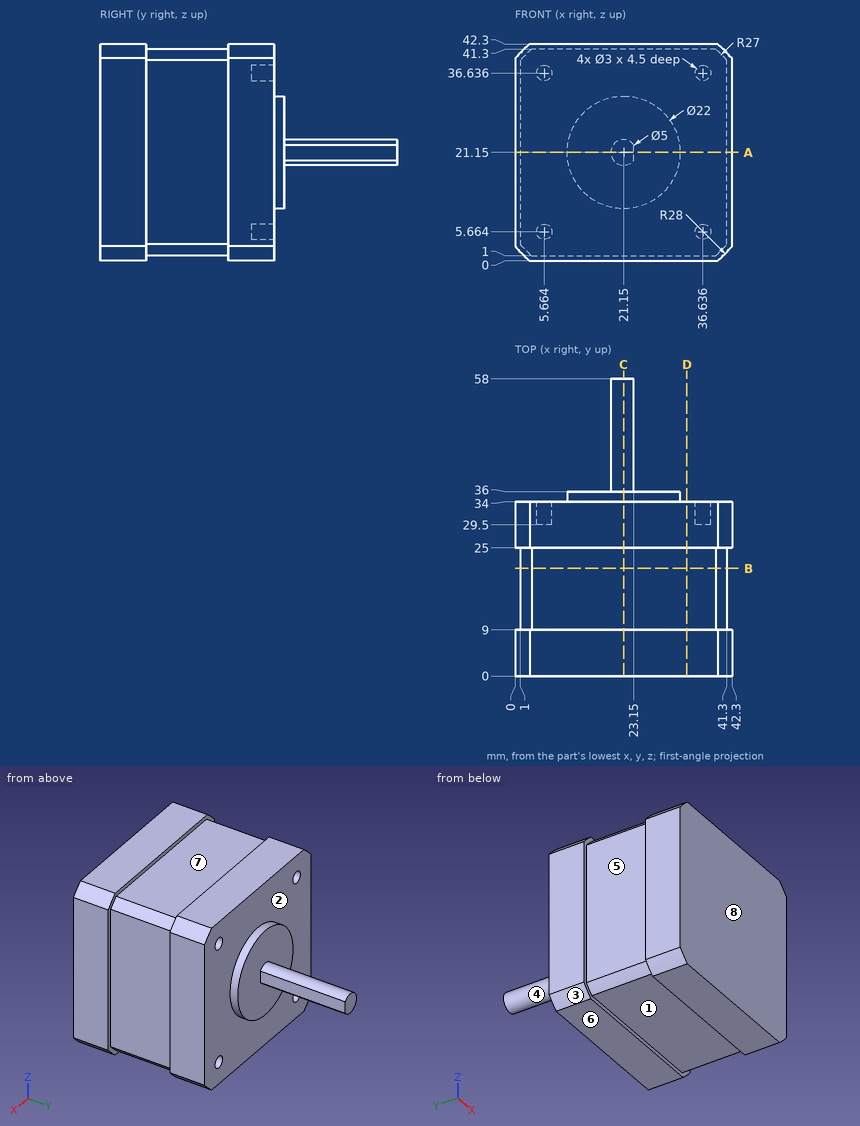
Job drawing, mm, ordinate dimensions from the low corner. One solid piece. A direction names the side the tool comes from. Give positions to 0.01 mm unless a question says otherwise; leave off trailing zeros. Loops run counter-clockwise (first coordinate to the right, second up) from the corner with the lowest first, then second, coordinate; pieces in that order, holes last.
Item 1: Slice it at D-D, the plane x = 33.5. List the corners of the cut face in (y, z), and give its area (3 significant figures).
Answers follow:
outline: (0, 0) - (9, 0) - (9, 1) - (25, 1) - (25, 0) - (34, 0) - (34, 42.3) - (25, 42.3) - (25, 41.3) - (9, 41.3) - (9, 42.3) - (0, 42.3) - close
area: 1,410 mm2
Item 2: Which spindle directions (+Z, -Z, +X, -X, +Y, -Y) get a long thin tool onto all of the face, cutting with end or side? Do the marked faces 4, 5, 6, 7 and 8. Say none if no direction does.
Answers follow:
face 4: +Y
face 5: +Z, -Z, -X
face 6: -Z, +X, -X, +Y, -Y
face 7: +Z, +X, -X
face 8: +Z, -Z, +X, -X, -Y
Item 3: Flat gauge pins, fed straight in: pin 1 (0.9 mm diameter, centred on x = 6, z = 5, fed in from +Y); pin 2 (3.5 mm diameter, centred on x = 36.64, z = 5.66, fed in from +Y); pin 3 (2.5 mm diameter, centred on y = 45.5, z = 21.5, fed in from +X). Where does each tip first touch, or does it go through?
Answers follow:
pin 1: stops at y = 29.5
pin 2: stops at y = 34
pin 3: stops at x = 23.15
Item 4: Drill centre lines: line 1 (Y direction, x = 24.5, z = 38); line 2 (X direction, y = 33.5, z = 5); line 3 (X direction, y = 11, z = 33.5). Where is each one in solid material? Low to high.
Answers follow:
line 1: y = 0 to 34
line 2: x = 0 to 4.32, 7.01 to 35.29, 37.98 to 42.3
line 3: x = 1 to 41.3
Item 5: Slice it at C-C, the plane x = 21.15. List the corners of the cut face in (y, z), and give its area (3 significant figures).
Answers follow:
outline: (0, 0) - (9, 0) - (9, 1) - (25, 1) - (25, 0) - (34, 0) - (34, 10.15) - (36, 10.15) - (36, 18.65) - (58, 18.65) - (58, 23.65) - (36, 23.65) - (36, 32.15) - (34, 32.15) - (34, 42.3) - (25, 42.3) - (25, 41.3) - (9, 41.3) - (9, 42.3) - (0, 42.3) - close
area: 1,560 mm2
Item 6: Slice it at B-B, the plane y = 21. List the corners of the cut face in (x, z).
Answers follow:
outline: (1, 3.18) arc R27 ccw to (3.18, 1) - (39.12, 1) arc R27 ccw to (41.3, 3.18) - (41.3, 39.12) arc R27 ccw to (39.12, 41.3) - (3.18, 41.3) arc R27 ccw to (1, 39.12) - close
Item 7: Pull direction Y, two halves, no side cores. Call the marked faces 1, 2 and 3: released by +Y, released by -Y, zero draft, split by the parting line, or undercut.
Answers follow:
face 1: undercut
face 2: released by +Y
face 3: zero draft
Item 8: Slice it at A-A, the plane z = 21.15. List the corners of the cut face in (x, y).
Answers follow:
outline: (0, 0) - (42.3, 0) - (42.3, 9) - (41.3, 9) - (41.3, 25) - (42.3, 25) - (42.3, 34) - (32.15, 34) - (32.15, 36) - (23.15, 36) - (23.15, 58) - (18.65, 58) - (18.65, 36) - (10.15, 36) - (10.15, 34) - (0, 34) - (0, 25) - (1, 25) - (1, 9) - (0, 9) - close
